Geometry: see drawing. Coordinates: mm, zero at the bounding-box minimum. Coordinates: 2 decimals unless noted, no trailing zeros. Order: outer loops, then holes, each group sorted by start corner. A loop starts at its lowest first (then second) coordinate and runs counter-clockwise, first axis right, second up.
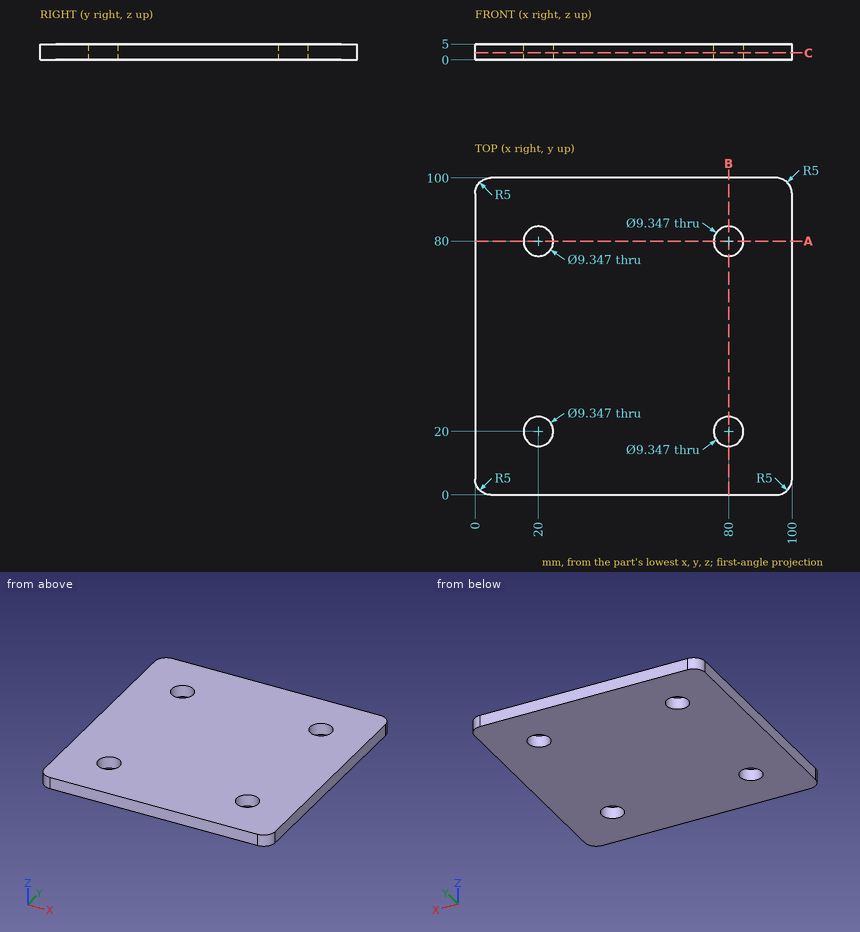
Q1. Section query C-C on z = 2.2. Output: boundary loops of the cut face in (x, y), plus the area to 3 significant figures.
Solutions:
outline: (0, 5) arc R5 ccw to (5, 0) - (95, 0) arc R5 ccw to (100, 5) - (100, 95) arc R5 ccw to (95, 100) - (5, 100) arc R5 ccw to (0, 95) - close; hole circle Ø9.35 at (20, 20); hole circle Ø9.35 at (20, 80); hole circle Ø9.35 at (80, 20); hole circle Ø9.35 at (80, 80)
area: 9,700 mm2
Q2. Section query A-A on y = 80. Output: boundary loops of the cut face in (x, z), plus the area to 3 significant figures.
Solutions:
outline: (0, 0) - (15.33, 0) - (15.33, 5) - (0, 5) - close; (24.67, 0) - (75.33, 0) - (75.33, 5) - (24.67, 5) - close; (84.67, 0) - (100, 0) - (100, 5) - (84.67, 5) - close
area: 407 mm2
Q3. Material intervals for line 1 along Y through (x, z) = (20, 2.95); line 2 along Y through (x, z) = (79.5, 0.45); line 3 along X through (y, z) = (84, 2.15), sorted ascending.
Solutions:
line 1: y = 0 to 15.33, 24.67 to 75.33, 84.67 to 100
line 2: y = 0 to 15.35, 24.65 to 75.35, 84.65 to 100
line 3: x = 0 to 17.58, 22.42 to 77.58, 82.42 to 100
